```python
from build123d import *

# Parameters (mm, degrees)
SKETCH1_W            = 17.92
SKETCH1_H            = 22.86
BOSS_EXTRUDE1_DEPTH  = 0.825
SKETCH3_R            = 0.5
CUT_EXTRUDE1_DEPTH   = 15.546722139
LPATTERN1_COUNT      = 8
LPATTERN1_PITCH      = 2.54
LPATTERN1_COUNT_DIR2 = 2
LPATTERN1_PITCH_DIR2 = 12.84
SKETCH4_W            = 18.95
SKETCH4_H            = 24
SKETCH4_W_2          = 14.95
SKETCH4_H_2          = 20
CUT_EXTRUDE2_DEPTH   = 15.616736982
FILLET1_R            = 1


with BuildPart() as part:
    # Sketch1 → Boss-Extrude1 (new, symmetric)
    with BuildSketch(Plane(origin=(0, 0, 0), x_dir=(1, 0, 0), z_dir=(0, 1, 0))):
        Rectangle(SKETCH1_W, SKETCH1_H)
    extrude(amount=BOSS_EXTRUDE1_DEPTH, both=True)

    # Sketch3 → Cut-Extrude1 (cut, symmetric)
    with BuildSketch(Plane(origin=(0, 0, 0), x_dir=(1, 0, 0), z_dir=(0, 1, 0))):
        with Locations(Location((-6.42, -8.89, 0), (0, 0, 270))):
            Circle(SKETCH3_R)
    cut_extrude1 = extrude(amount=CUT_EXTRUDE1_DEPTH, both=True, mode=Mode.SUBTRACT)

    # LPattern1: Cut-Extrude1 8 × 2
    with Locations(*[(j * LPATTERN1_PITCH_DIR2, 0, -i * LPATTERN1_PITCH) for i in range(LPATTERN1_COUNT) for j in range(LPATTERN1_COUNT_DIR2) if (i, j) != (0, 0)]):
        add(cut_extrude1, mode=Mode.SUBTRACT)

    # Sketch4 → Cut-Extrude2 (cut, through all)
    with BuildSketch(Plane(origin=(0, 0.825, 0), x_dir=(1, 0, 0), z_dir=(0, 1, 0))):
        with Locations((0, -0.28)):
            Rectangle(SKETCH4_W, SKETCH4_H)
        with Locations((0, -0.28)):
            Rectangle(SKETCH4_W_2, SKETCH4_H_2, mode=Mode.SUBTRACT)
    extrude(amount=-CUT_EXTRUDE2_DEPTH, mode=Mode.SUBTRACT)

    # Fillet1
    fillet1_edges = [part.edges().sort_by_distance(p)[0] for p in [
        (-7.475, 0, -9.72),
        (7.475, 0, -9.72),
        (7.475, 0, 10.28),
        (-7.475, 0, 10.28),
    ]]
    fillet(fillet1_edges, radius=FILLET1_R)


solid = part.part
```
CAD build for the part. Positions are in the model's coordinates, mm. Coordinates: 2 decimals unless noted, no trailing zeros. Order: outer loops, then holes, each group sorted by start corner. A loop starts at its lowest first (then second) coordinate and runs counter-clockwise, first axis right, second up. Notation, with made-up numbers: (70, 87.25) - (128, 87.25) arc R14 cw to (128, 98.25) - close; hole circle Ø6 at (32.25, -21.75). An arc over 180 degrees is marked (long way). Use a Markdown table: item, result. Add a question column.
(1) Saw through at B-B (y = -0.3). Count the separate pieces of the cut face and the enclosed holes in it, then the cut area to 3 significant figures.
(2) Saw through at A-A (z = 6.35). Give the cut face in (x, y) (3 decimals), then the cut area to 3 significant figures.
(3) Drill centre lines: line 1 along X through (y, z) = (0.3, 6.35) (3 decimals); line 2 along X through (y, z) = (0.2, -1.5) (3 decimals). Where is each one in solid material? Low to high. Write a range as [from, to].
Solved:
| question | item | result |
|---|---|---|
| 1 | separate pieces | 1 |
| 1 | enclosed holes | 16 |
| 1 | area | 286 mm² |
| 2 | outline | (-7.475, -0.825) - (-6.92, -0.825) - (-6.92, 0.825) - (-7.475, 0.825) - close; (-5.92, -0.825) - (5.92, -0.825) - (5.92, 0.825) - (-5.92, 0.825) - close; (6.92, -0.825) - (7.475, -0.825) - (7.475, 0.825) - (6.92, 0.825) - close |
| 2 | area | 21.4 mm² |
| 3 | line 1 | x = [-7.475, -6.92], [-5.92, 5.92], [6.92, 7.475] |
| 3 | line 2 | x = [-7.475, -6.864], [-5.976, 5.976], [6.864, 7.475] |
